Autodesk Inventor part; units mm, degrees
ref_plane "Arbeitsebene1" through (0, 0, 32) normal (0, 0, 1) x (1, 0, 0)
ref_plane "YZ Plane" through (0, 0, 0) normal (1, 0, 0) x (0, 1, 0)
ref_plane "XZ Plane" through (0, 0, 0) normal (0, 1, 0) x (-1, 0, 0)
sketch "Skizze1" plane through (0, 0, 0) normal (0, 0, 1) x (1, 0, 0)
  line L0 (-18, -13) -> (18, -13)
  line L1 (18, -13) -> (18, 13)
  line L2 (18, 13) -> (-18, 13)
  line L3 (-18, 13) -> (-18, -13)
extrude "Extrusion1" add sketch "Skizze1" along normal blind 32
sketch "Skizze2" plane through (0, 0, 0) normal (0, 0, 1) x (1, 0, 0)
  circle A0 centre (0, 0) radius 2.5
extrude "Extrusion2" cut sketch "Skizze2" along normal blind 4.2
sketch "Skizze3" plane through (0, 0, 0) normal (0, 0, 1) x (1, 0, 0)
  line L0 (3.3, -1) -> (5.8, -1)
  line L1 (5.8, -1) -> (5.8, 1)
  line L2 (5.8, 1) -> (3.3, 1)
  line L3 (3.3, 1) -> (3.3, -1)
extrude "Extrusion3" cut sketch "Skizze3" along normal blind 4.2
sketch "Skizze4" plane through (0, 0, 0) normal (0, 0, 1) x (1, 0, 0)
  line L0 (-5.8, -1) -> (-3.3, -1)
  line L1 (-3.3, -1) -> (-3.3, 1)
  line L2 (-3.3, 1) -> (-5.8, 1)
  line L3 (-5.8, 1) -> (-5.8, -1)
extrude "Extrusion4" cut sketch "Skizze4" along normal blind 4.2
sketch "Skizze5" plane through (0, 0, 0) normal (0, 0, 1) x (1, 0, 0)
  line L0 (-1, 3.3) -> (1, 3.3)
  line L1 (1, 3.3) -> (1, 5.8)
  line L2 (1, 5.8) -> (-1, 5.8)
  line L3 (-1, 5.8) -> (-1, 3.3)
extrude "Extrusion5" cut sketch "Skizze5" along normal blind 4.2
sketch "Skizze6" plane through (0, 0, 0) normal (0, 0, 1) x (1, 0, 0)
  line L0 (-1, -5.8) -> (1, -5.8)
  line L1 (1, -5.8) -> (1, -3.3)
  line L2 (1, -3.3) -> (-1, -3.3)
  line L3 (-1, -3.3) -> (-1, -5.8)
extrude "Extrusion6" cut sketch "Skizze6" along normal blind 4.2
sketch "Skizze7" plane through (0, 0, 0) normal (0, 0, 1) x (1, 0, 0)
  circle A0 centre (-14.5, 0) radius 1.4
extrude "Extrusion7" cut sketch "Skizze7" along normal blind 32.2
sketch "Skizze8" plane through (0, 0, 0) normal (0, 0, 1) x (1, 0, 0)
  circle A0 centre (14.5, 0) radius 1.4
extrude "Extrusion8" cut sketch "Skizze8" along normal blind 32.2
ref_plane "Arbeitsebene1" through (0, 0, 32) normal (0, 0, 1) x (1, 0, 0)
sketch "Skizze9" plane through (0, 0, 32) normal (0, 0, 1) x (1, 0, 0)
  circle A0 centre (0, 0) radius 11
extrude "Extrusion9" cut sketch "Skizze9" against normal blind 28
sketch "Skizze10" plane through (0, 0, 0) normal (0, 1, 0) x (-1, 0, 0)
  line L0 (-8, 5) -> (8, 5)
  line L1 (8, 5) -> (8, 27)
  line L2 (8, 27) -> (-8, 27)
  line L3 (-8, 27) -> (-8, 5)
extrude "Extrusion10" cut sketch "Skizze10" along normal mid plane 30
properties part number "Motorblock_N20"
Input: part model. Units: mm. Frame: model coordinates. A direction names the side the tool comes from. Round coordinates to 2 decimals unless told otherwise and drop trailing zeros. Write each loop counter-clockwise with the first axis right and the second up, starting at its lowest first coordinate (ties: lowest second). Pieces come first, ordered by that corner, then holes.
1) Reachability of faces 1 (the flat face through (0, -12, 5)), 2 (the flat face through (-1, -5, 2)), 3 (the flat face through (18, 0, 16)) from +Z, -Z, +X, -X, +Y, -Y: full face, straight path, thin tool, end or side. Return the list, or none.
2) Draft query along Z for faces 4 (the flat face through (-0.3, -11.4, 32)), 5 (the cylindrical face through (-0.54, 2.44, 1.97)), 6 (the flat face through (0, 3, 0)), 7 (the flat face through (0.1, 11.4, 5)). Return one class per face: pulls with the +Z half, pulls with the -Z half, needs draft (parallel to the pull), parting line crosses it, or undercut.
3) Cut plane B-B (x = 0). Return the cut outline in (y, z).
4) Cut plane D-D (x = -14.5). Return the cut outline in (y, z).
5) Cut plane C-C (y = 0). Return the cut outline in (x, z), then the cut area to 3 significant figures.
6) Ray query, L1, parallel to Y at x = 0, z = 1.3; L2, parallel to X at y = -9.5, z = 17.5; L3, parallel to Z at x = -7.5, y = -7.25. Return the intervals inside material, ascending.
7) Cut plane A-A (z = 16.5). Return the cut outline in (x, y), then the cut area to 3 significant figures.
Geometry says:
1. face 1: +Y, -Y
1. face 2: +Z, -Z
1. face 3: +Z, -Z, +X, +Y, -Y
2. face 4: pulls with the +Z half
2. face 5: needs draft
2. face 6: pulls with the -Z half
2. face 7: undercut
3. outline: (-13, 0) - (-5.8, 0) - (-5.8, 4) - (-11, 4) - (-11, 5) - (-13, 5) - close; (-13, 27) - (-11, 27) - (-11, 32) - (-13, 32) - close; (-3.3, 0) - (-2.5, 0) - (-2.5, 4) - (-3.3, 4) - close; (2.5, 0) - (3.3, 0) - (3.3, 4) - (2.5, 4) - close; (5.8, 0) - (13, 0) - (13, 5) - (11, 5) - (11, 4) - (5.8, 4) - close; (11, 27) - (13, 27) - (13, 32) - (11, 32) - close
4. outline: (-13, 0) - (-1.4, 0) - (-1.4, 32) - (-13, 32) - close; (1.4, 0) - (13, 0) - (13, 32) - (1.4, 32) - close
5. outline: (-18, 0) - (-15.9, 0) - (-15.9, 32) - (-18, 32) - close; (-13.1, 0) - (-5.8, 0) - (-5.8, 4) - (-11, 4) - (-11, 32) - (-13.1, 32) - close; (-3.3, 0) - (-2.5, 0) - (-2.5, 4) - (-3.3, 4) - close; (2.5, 0) - (3.3, 0) - (3.3, 4) - (2.5, 4) - close; (5.8, 0) - (13.1, 0) - (13.1, 32) - (11, 32) - (11, 4) - (5.8, 4) - close; (15.9, 0) - (18, 0) - (18, 32) - (15.9, 32) - close
5. area: 317 mm2
6. L1: y = -13 to -5.8, -3.3 to -2.5, 2.5 to 3.3, 5.8 to 13
6. L2: x = -18 to -8, 8 to 18
6. L3: z = 0 to 4
7. outline: (-18, -13) - (-8, -13) - (-8, -7.55) arc R11 cw to (-8, 7.55) - (-8, 13) - (-18, 13) - close; (8, -13) - (18, -13) - (18, 13) - (8, 13) - (8, 7.55) arc R11 cw to (8, -7.55) - close; hole circle Ø2.8 at (-14.5, 0); hole circle Ø2.8 at (14.5, 0)
7. area: 445 mm2
